Check sheet for the modelled part. Datum: model origin and axes. Units: mm. A direction names the side the tool comes from. Give positions to 0.01 mm unless a question says otherwise; leave off trailing zeros. Loops run counter-clockwise (first coordinate to the right, second up) from the corner with the lowest first, then second, coordinate; pieces in that order, holes last. Notation, with made-up numbers: (42, -17.75) - (54, -17.75) arc R13 ccw to (54, -13.75) - close; hole circle Ø5 at (52, 16). An arc over 180 degrees is marked (long way). Answer in a Markdown table with one row per item. Add a question column.
(1) Sectioned sample at B-B on x = -58.5. Enter the section's corners in (y, z).
(2) Set-up check for faces 5 (the face through (-3, 77, -76.2)), 6 (the face through (-3, 76, -120.595)): record each of +Z, -Z, +X, -X, +Y, -Y from which the full face is reachable in a straight line by a thin tool's end or side.
(3) Draft check along Z on faces 1 (the face through (-3, 76, -82.605)), 2 (the face through (-15, 50.8, -122)), 3 (the face through (-3, 77, -127)), 4 (the face through (188.69, 75.84, -78.11)). Enter one of: released by +Z, released by -Z, zero draft, split by the parting line, or undercut.
(4) Sectioned sample at A-A on z = -106.5. Enter the section's corners in (x, y).
(5) Thickness scan on L1, parallel to X at y = 87.5, z = -105; L2, parallel to Z at x = 170, y = 57. Record the ranges inside material, lowest first.
(6) Sectioned sample at C-C on y = 71. Enter the section's corners in (x, z) (3 decimals), then the cut area to 3 significant figures.
from build123d import *

# Parameters (mm, degrees)
F0_W     = 381
F0_H     = 50.8
F1_DEPTH = 50.8
F2_R     = 6.35
F3_R     = 5.08
F5_W     = 368.3
F5_H     = 37.989244
F6_DEPTH = 50.8
F7_R     = 3.175


with BuildPart() as f1:
    # F0 (on Front) → F1 (new body)
    with BuildSketch(Plane.XZ):
        Rectangle(F0_W, F0_H)
    extrude(amount=F1_DEPTH)

    # F2
    f2_edges = [f1.edges().sort_by_distance(p)[0] for p in [
        (190.5, -25.4, 25.4),
    ]]
    fillet(f2_edges, radius=F2_R)

    # F3
    f3_edges = [f1.edges().sort_by_distance(p)[0] for p in [
        (190.5, -25.4, -25.4),
        (-190.5, -25.4, 25.4),
        (-190.5, -25.4, -25.4),
    ]]
    fillet(f3_edges, radius=F3_R)


with BuildPart() as f1_1:
    # F4: moved
    add(f1.part.moved(Location((0, 50.8, 0))))

    # F5 (on Front) → F6 (cut)
    with BuildSketch(Plane.XZ):
        Rectangle(F5_W, F5_H)
    extrude(amount=-F6_DEPTH, mode=Mode.SUBTRACT)

    # F7
    f7_edges = [f1_1.edges().sort_by_distance(p)[0] for p in [
        (184.15, 25.4, -18.994622),
        (184.15, 25.4, 18.994622),
        (-184.15, 25.4, 18.994622),
        (-184.15, 25.4, -18.994622),
    ]]
    fillet(f7_edges, radius=F7_R)


with BuildPart() as f1_2:
    # F8: moved
    add(f1_1.part.moved(Location((0, 50.8, 0))))


with BuildPart() as f1_3:
    # F9: moved
    add(f1_2.part.moved(Location((0, 0, -101.6))))


solid = f1_3.part
Reply:
| question | item | result |
|---|---|---|
| 1 | outline | (50.8, -127) - (101.6, -127) - (101.6, -120.59) - (50.8, -120.59) - close; (50.8, -82.61) - (101.6, -82.61) - (101.6, -76.2) - (50.8, -76.2) - close |
| 2 | face 5 | +Z, +X, -X, +Y, -Y |
| 2 | face 6 | +Y, -Y |
| 3 | face 1 | undercut |
| 3 | face 2 | zero draft |
| 3 | face 3 | released by -Z |
| 3 | face 4 | released by +Z |
| 4 | outline | (-190.5, 50.8) - (-184.15, 50.8) - (-184.15, 101.6) - (-190.5, 101.6) - close; (184.15, 50.8) - (190.5, 50.8) - (190.5, 101.6) - (184.15, 101.6) - close |
| 5 | L1 | -190.5 to -184.15, 184.15 to 190.5 |
| 5 | L2 | -127 to -120.59, -82.61 to -76.2 |
| 6 | outline | (-190.5, -121.92) arc R5.08 ccw to (-185.42, -127) - (185.42, -127) arc R5.08 ccw to (190.5, -121.92) - (190.5, -82.55) arc R6.35 ccw to (184.15, -76.2) - (-185.42, -76.2) arc R5.08 ccw to (-190.5, -81.28) - close; hole (-184.15, -117.42) arc R3.175 ccw to (-180.975, -120.595) - (180.975, -120.595) arc R3.175 ccw to (184.15, -117.42) - (184.15, -85.78) arc R3.175 ccw to (180.975, -82.605) - (-180.975, -82.605) arc R3.175 ccw to (-184.15, -85.78) - close |
| 6 | area | 5,350 mm^2 |
